Verification items for the finished model (mm, model axes). Face numbers are marked on the shaded views. A direction names the side the tool comes from. Round coordinates to 2 decimals unless told otherwise and drop trailing zeros. Write each loop counter-clockwise with the first axis right and the second up, starting at its lowest first coordinate (ties: lowest second). Pieces come first, ordered by that corner, then holes. Notation, with made-up numbers: M 51.25,18.5 L 71.25,18.5 A9 ccw 71.25,31.5 Z; hole C 42.5,-35.75 d6. An arc over 180 degrees is marked long. Write each question's results on one line, items separated by ' | '.
from build123d import *

# Parameters (mm, degrees)
SKETCH1_R           = 4
BOSS_EXTRUDE2_DEPTH = 30
SKETCH3_R           = 2.5
CUT_EXTRUDE1_DEPTH  = 12
SKETCH4_R           = 2.16
CUT_EXTRUDE2_DEPTH  = 31
SKETCH10_OUTSIDE_W  = 16.412
SKETCH10_OUTSIDE_H  = 16.412
SKETCH10_OUTSIDE_R  = 3.556
CUT_EXTRUDE3_DEPTH  = 15
SKETCH18_OUTSIDE_W  = 16.412
SKETCH18_OUTSIDE_H  = 16.412
SKETCH18_OUTSIDE_R  = 3.225571995
CUT_EXTRUDE4_DEPTH  = 7.5


with BuildPart() as part:
    # Sketch1 → Boss-Extrude2 (new body)
    with BuildSketch(Plane(origin=(0, 0, 0), x_dir=(0, 0, -1), z_dir=(1, 0, 0))):
        Circle(SKETCH1_R)
    extrude(amount=BOSS_EXTRUDE2_DEPTH)

    # Sketch3 → Cut-Extrude1 (cut)
    with BuildSketch(Plane.ZY):
        Circle(SKETCH3_R)
    extrude(amount=-CUT_EXTRUDE1_DEPTH, mode=Mode.SUBTRACT)

    # Sketch4 → Cut-Extrude2 (cut, through all)
    with BuildSketch(Plane(origin=(30, 0, 0), x_dir=(0, 0, -1), z_dir=(1, 0, 0))):
        Circle(SKETCH4_R)
    extrude(amount=-CUT_EXTRUDE2_DEPTH, mode=Mode.SUBTRACT)

    # Sketch10 outside → Cut-Extrude3 (cut)
    with BuildSketch(Plane(origin=(30, 0, 0), x_dir=(0, 0, -1), z_dir=(1, 0, 0))):
        Rectangle(SKETCH10_OUTSIDE_W, SKETCH10_OUTSIDE_H)
        Circle(SKETCH10_OUTSIDE_R, mode=Mode.SUBTRACT)
    extrude(amount=-CUT_EXTRUDE3_DEPTH, mode=Mode.SUBTRACT)

    # Sketch18 outside → Cut-Extrude4 (cut)
    with BuildSketch(Plane(origin=(15, 0, 0), x_dir=(0, 0, -1), z_dir=(1, 0, 0))):
        Rectangle(SKETCH18_OUTSIDE_W, SKETCH18_OUTSIDE_H)
        Circle(SKETCH18_OUTSIDE_R, mode=Mode.SUBTRACT)
    extrude(amount=CUT_EXTRUDE4_DEPTH, mode=Mode.SUBTRACT)

    # Sketch17 → Cut-Revolve1 (revolve, cut)
    with BuildSketch(Plane.XY):
        Polygon((28.84073404, 3.90926596), (30, 2.75), (28.84073404, 1.59073404), (31.351449917, 1.59073404), (31.351449917, 3.90926596), align=None)
    revolve(axis=Axis((12, 0, 0), (1, 0, 0)), mode=Mode.SUBTRACT)


solid = part.part
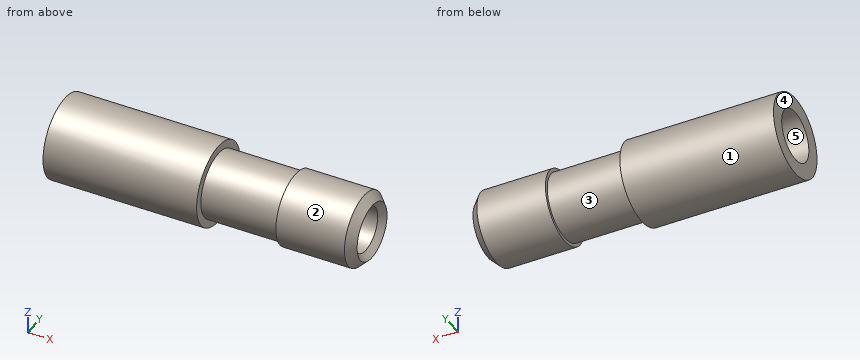
1) Material ranges on line 1 (Z direction, x = 25, y = 0); line 2 (Y direction, x = 4.5, z = 0); line 3 (Y direction, x = 22, z = 0), recorded low to high. Write a range as [from, to].
Calculated:
line 1: z = [-3.56, -2.16], [2.16, 3.56] | line 2: y = [-4, -2.5], [2.5, 4] | line 3: y = [-3.23, -2.16], [2.16, 3.23]
2) Access from +Z, -Z, +X, -X, +Y, -Y to the whole of each face (thin tool, end or side, straight path). Record for the marked faces 1 and 2.
Calculated:
face 1: +X, -X | face 2: +X
3) Depth check by flat-ended pin: P1, Ø3, axis at x = 18.5, z = -2.5, coming from the -Y side. Enter the tip coordinate at first touch or a pass-through.
Calculated:
P1: stops at y = -3.07
4) Draft check along Y on the marked faces 3, 4 and 5. Enter one of: pulls with the +Y half, pulls with the -Y half, needs draft (parallel to the pull), parting line crosses it, or undercut.
Calculated:
face 3: parting line crosses it | face 4: needs draft | face 5: undercut
5) Sectioned sample at C-C, the plane x = 14.5. Record the cut outline in (y, z), and give its area (3 significant figures).
Calculated:
outline: C 0,0 d8; hole C 0,0 d4.32 | area: 35.6 mm²
6) Sectioned sample at A-A, the plane y = 0. Record the cut outline in (x, z).
Calculated:
outline: M 0,-4 L 15,-4 L 15,-3.23 L 22.5,-3.23 L 22.5,-3.56 L 29.19,-3.56 L 30,-2.75 L 29.41,-2.16 L 12,-2.16 L 12,-2.5 L 0,-2.5 Z; M 0,2.5 L 12,2.5 L 12,2.16 L 29.41,2.16 L 30,2.75 L 29.19,3.56 L 22.5,3.56 L 22.5,3.23 L 15,3.23 L 15,4 L 0,4 Z
7) Sectioned sample at D-D, the plane x = 2. Record the cut outline in (y, z).
Calculated:
outline: C 0,0 d8; hole C 0,0 d5
